Autodesk Inventor part; units mm, degrees
ref_plane "YZ Plane" through (0, 0, 0) normal (1, 0, 0) x (0, 1, 0)
ref_plane "XZ Plane" through (0, 0, 0) normal (0, 1, 0) x (-1, 0, 0)
ref_plane "XY Plane" through (0, 0, 0) normal (0, 0, 1) x (1, 0, 0)
sketch "Sketch1" plane through (0, 0, 0) normal (0, 0, 1) x (1, 0, 0)
  line L0 (-15.875, -12.7) -> (15.875, -12.7)
  line L1 (15.875, -12.7) -> (15.875, 12.7)
  line L2 (15.875, 12.7) -> (-15.875, 12.7)
  line L3 (-15.875, 12.7) -> (-15.875, -12.7)
  line L4 (-15.875, -12.7) -> (15.875, 12.7) construction
  line L5 (15.875, -12.7) -> (-15.875, 12.7) construction
  point P0 (0, 0)
  dimension "d0" = 31.75
  dimension "d1" = 25.4
extrude "Extrusion1" add sketch "Sketch1" against normal blind 12.7
sketch "Sketch2" plane through (-15.875, -12.7, 0) normal (-1, 0, 0) x (0, 0, 1)
  line L0 (-12.7, 0) -> (-12.7, 25.4) construction
  line L1 (0, 25.4) -> (0, 0) construction
  line L2 (-12.7, 25.4) -> (0, 0) construction
  line L3 (0, 25.4) -> (-12.7, 0) construction
  circle A0 centre (-6.35, 12.7) radius 3.683
  point P0 (0, 12.7)
  dimension "d4" = 7.366
extrude "Extrusion2" cut sketch "Sketch2" against normal blind 9.525
sketch "Sketch3" plane through (0, 0, 0) normal (0, 0, 1) x (1, 0, 0)
  circle A0 centre (0, 0) radius 5.2705
  dimension "d7" = 10.541
extrude "Extrusion3" cut sketch "Sketch3" against normal through all
properties part number "tieRod"
Geometry: final body of the model. Coordinates: model frame, mm. A direction names the side the tool comes from. Coordinates: 2 decimals unless noted, no trailing zeros. Order: outer loops, then holes, each group sorted by start corner. A loop starts at its lowest first (then second) coordinate and runs counter-clockwise, first axis right, second up. Notation, with made-up numbers: (27, 82) -> (43, 82) arc R27 cw to (43, 98) -> close; hole circle Ø7 at (3.25, -11). An arc over 180 degrees is marked (long way). Answer in a Markdown table with one row per item.
Item 1: Section D-D on x = 0. Output: boundary loops of the cut face in (y, z), plus the area to 3 significant figures.
Return value:
| item | result |
|---|---|
| outline | (-12.7, -12.7) -> (-5.27, -12.7) -> (-5.27, 0) -> (-12.7, 0) -> close; (5.27, -12.7) -> (12.7, -12.7) -> (12.7, 0) -> (5.27, 0) -> close |
| area | 189 mm² |
Item 2: Ray query, L1, parallel to Y at x = 0, z = -4.75; L2, parallel to Y at x = -11.25, z = -6.35; L3, parallel to X at y = 3, z = -11.25 (3 decimals). Return the intervals inside material, ascending.
Return value:
| item | result |
|---|---|
| L1 | y = -12.7 to -5.27, 5.27 to 12.7 |
| L2 | y = -12.7 to -3.68, 3.68 to 12.7 |
| L3 | x = -15.875 to -4.333, 4.333 to 15.875 |
Item 3: Section C-C on x = -7.5. Output: boundary loops of the cut face in (y, z), plus the area to 3 significant figures.
Return value:
| item | result |
|---|---|
| outline | (-12.7, -12.7) -> (12.7, -12.7) -> (12.7, 0) -> (-12.7, 0) -> close; hole circle Ø7.37 at (0, -6.35) |
| area | 280 mm² |
Item 4: Draft query along X for faces 3 (the flat face through (15.875, 0, -6)), 4 (the flat face through (-0.2, -5.5, -12.7)), 5 (the cylindrical face through (5.03, 1.58, -6.26)). Return one class per face: released by +X, released by -X, zero draft, split by the parting line, or undercut.
Return value:
| item | result |
|---|---|
| face 3 | released by +X |
| face 4 | zero draft |
| face 5 | undercut |
Item 5: Access query for faces 1 (the flat face through (-0.2, -5.5, 0)), 2 (the flat face through (-6.35, 0, -6)). Directions: +Z, -Z, +X, -X, +Y, -Y. A direction counts if a zero-diameter tool reaches every point of the face in a straight line with its end or side. Return the directions, or none.
Return value:
| item | result |
|---|---|
| face 1 | +Z, +X, -X, +Y, -Y |
| face 2 | -X |
Item 6: Contact query for flat-ended pins moving along their axis: P1, Ø3, axis at x = -1, y = 3.5, coming from the -Z side; P2, Ø2, axis at y = 1.5, z = -7.5, coming from the -X side. Output: stop coordinate, or through.
Return value:
| item | result |
|---|---|
| P1 | passes through |
| P2 | stops at x = -6.35 |
